The listing builds one solid part. Answer for the finished solid, in the listing's coordinates (mm). Coordinates: 2 decimals unless noted, no trailing zeros. Loops run counter-clockwise (first coordinate to the right, second up) from the corner with the lowest first, then second, coordinate; pieces in that order, holes last. Notation, with made-up numbers: (-33, 11.5) - (24, 11.5) arc R28 cw to (24, 31.5) - close; hole circle Ø9 at (6.25, 8). An arc over 180 degrees is marked (long way). Put each result on its own line as item: value.
```python
from build123d import *

# Parameters (mm, degrees)
DODANIE_WYCI_GNI_CIE1_DEPTH = 2
ZAOKR_GLENIE1_R             = 1


with BuildPart() as part:
    # Szkic1 → Dodanie-wyciągnięcie1 (new body)
    with BuildSketch(Plane.XY):
        Polygon((35, 90), (15.738496678, 90), (0, 52.892860976), (14.054590176, 54.576767478), (0, 28.625581399), (11.064716979, 30.848994041), (0, 0), (30.019363734, 40.738188486), (16.772070835, 39.719165955), (33.803123901, 65.598770402), (18.399416714, 64.413869849), align=None)
    extrude(amount=DODANIE_WYCI_GNI_CIE1_DEPTH)

    # Zaokrąglenie1
    zaokr_glenie1_edges = [part.edges().sort_by_distance(p)[0] for p in [
        (5.532358489, 15.424497021, 0),
        (5.532358489, 29.73728772, 0),
        (7.027295088, 41.601174439, 0),
        (7.027295088, 53.734814227, 0),
        (7.869248339, 71.446430488, 0),
        (25.369248339, 90, 0),
        (26.699708357, 77.206934925, 0),
        (26.101270307, 65.006320126, 0),
        (25.287597368, 52.658968179, 0),
        (23.395717284, 40.228677221, 0),
        (15.009681867, 20.369094243, 0),
    ]]
    fillet(zaokr_glenie1_edges, radius=ZAOKR_GLENIE1_R)


solid = part.part
```
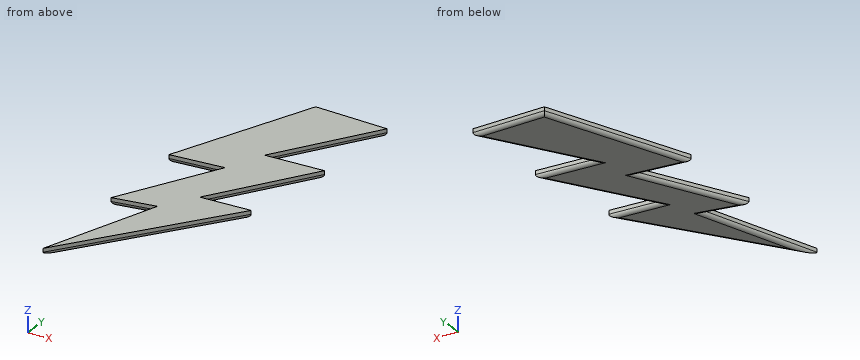
1) The part is cut by section A-A (z = 0.3). Give the vertices of the cut face in (x, y), and give its area (3 significant figures).
Found:
outline: (0.46, 53.24) - (14.57, 54.93) - (0.54, 29.03) - (11.5, 31.23) - (0.93, 1.74) - (29.42, 40.41) - (16.21, 39.39) - (33.24, 65.27) - (17.84, 64.08) - (34.47, 89.71) - (15.93, 89.71) - close
area: 1,190 mm^2
2) Straight lines are drawn through the part: L1, parallel to Y at x = 21, z = 0.8; L2, parallel to Y at x = 19.5, z = 1.05; L3, parallel to Y at x = 32, z = 0.55. For each, find the intervals that lie inside material, in ascending order. Write a range as [from, to].
Found:
L1: y = [28.53, 40.02], [46.18, 64.59], [68.46, 89.98]
L2: y = [26.46, 39.93], [43.86, 64.5], [66.11, 90]
L3: y = [63.05, 65.35], [85.57, 89.89]
3) The part is cut by section B-B (x = 9.5). State how many separate pieces and enclosed holes the cut face has, and give its area (3 significant figures).
Found:
separate pieces: 3
enclosed holes: 0
area: 98.5 mm^2
4) This flat-tipped pin is pushed along its axis until it touches: pin 1 (12 mm diameter, centred on x = 16, y = 14, fed in from +Z). Where does it stop, or does it pass through?
Found:
pin 1: stops at z = 2
